Here's the drawing with two shaded views (mm, measured from the low corner). I have some questions. Round coordinates to 2 decimals unless told otherwise and drop trailing zeros. Order: outer loops, then holes, each group sorted by start corner. A loop starts at its lowest first (then second) coordinate and runs counter-clockwise, first axis right, second up. Notation, with made-up numbers: (46.5, 76) - (90.5, 76) arc R21 cw to (90.5, 113) - close; hole circle Ø7 at (-16, 2.25). An arc over 180 degrees is marked (long way). One line per item, written item: value.
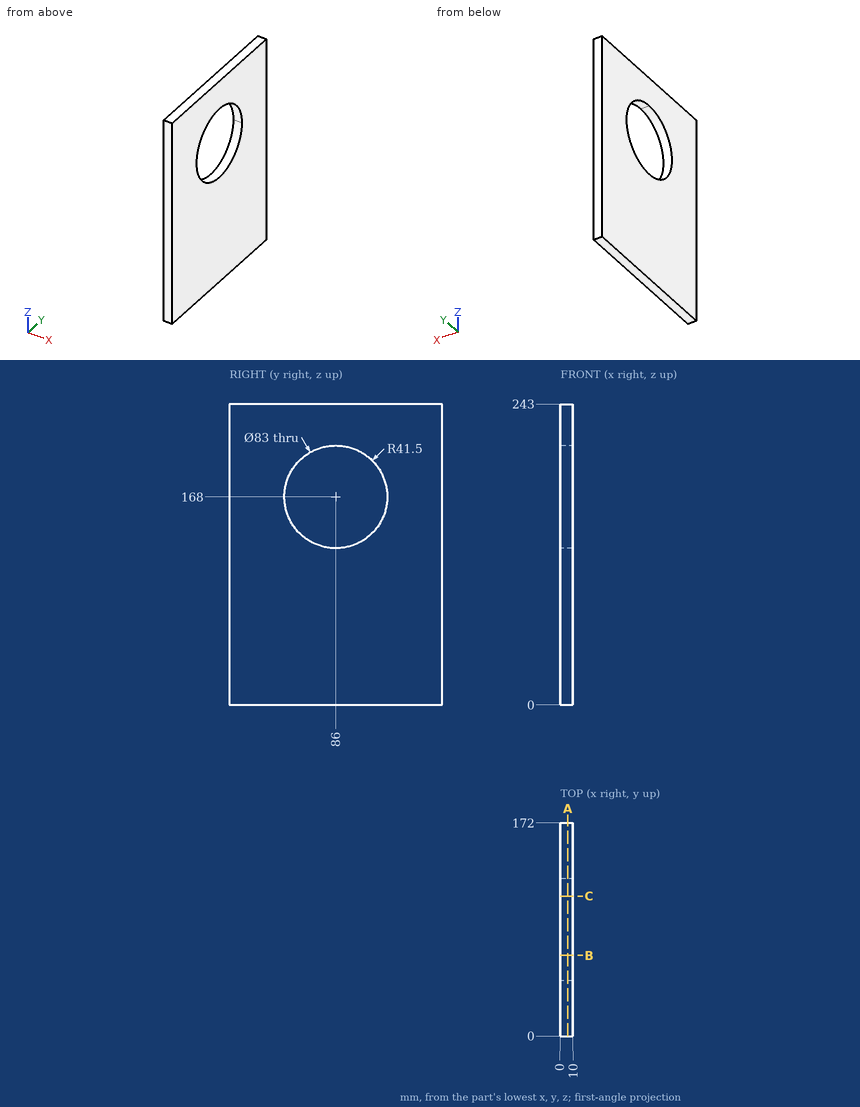
Q1. If we section it at C-C, the plane y = 113: Please give me the cut outline in (x, z), then the cut area to 3 significant figures.
Results list:
outline: (0, 0) - (10, 0) - (10, 136.48) - (0, 136.48) - close; (0, 199.52) - (10, 199.52) - (10, 243) - (0, 243) - close
area: 1,800 mm²
Q2. If we section it at B-B, the plane y = 65: Please give me the cut outline in (x, z), then the cut area to 3 significant figures.
Results list:
outline: (0, 0) - (10, 0) - (10, 132.21) - (0, 132.21) - close; (0, 203.79) - (10, 203.79) - (10, 243) - (0, 243) - close
area: 1,710 mm²
Q3. If I drill on line 1 along Z through (x, y) = (3.75, 86); line 2 along Y through (x, z) = (6.5, 168); line 3 along Y through (x, z) = (6, 166), over which ranges is the centre line in solid material (lowest first)?
Results list:
line 1: 0 to 126.5, 209.5 to 243
line 2: 0 to 44.5, 127.5 to 172
line 3: 0 to 44.55, 127.45 to 172
Q4. If we section it at A-A, the plane x = 6: Please give me the cut outline in (y, z).
Results list:
outline: (0, 0) - (172, 0) - (172, 243) - (0, 243) - close; hole (86, 209.5) arc R41.5 ccw (long way) to (127.5, 168) arc R41.5 ccw to start
Q5. Will this pin go through, and if not, where does the flat tip stop? pin 1 (5 mm diameter, centred on x = 3, z = 102.5, fed in from -Y).
Results list:
pin 1: y = 0
